Could you check a few things on this model? Use its own coordinates, in mm. Give positions to 0.01 mm unless a question says otherwise; leave off trailing zeros. Loops run counter-clockwise (first coordinate to the right, second up) from the corner with the lowest first, then second, coordinate; pieces in that order, holes last. Notation, with made-up numbers: M -22,77.5 L 13,77.5 A30 ccw 13,100.5 Z; hole C 59.25,71 d11. An arc over 180 degrees is marked long. Answer in a Markdown table with one row per item. Add a question column.
1. If we section it at D-D on x = -16.5: List the corners of the cut face in (y, z) for me.
2. If we section it at B-B on x = 0: List the corners of the cut face in (y, z) for me, then the cut area to 3 significant figures.
3. If we section it at A-A on z = 0: List the corners of the cut face in (x, y) for me.
4. If we section it at C-C on y = 1.6: Count the separate pieces of the cut face and the enclosed holes in it, then the cut area to 3 significant figures.
5. I need wall thicknesses on line 1 along Z through (x, y) = (0, 1.3); line 2 along Z through (x, y) = (-22.5, 0.95); line 3 along Z through (x, y) = (-7.5, 2). Which ranges of each line are inside material? Lowest first, please. Write a range as from..to.
6. I'm going to push flat-ended pins straight in: pin 1 Ø2 at (x, z) = (8.13, -22.27) entering from -Y; pin 2 Ø1 at (x, y) = (-11, 2.5) entering from -Z. Where does each tip first touch, or does it pass through?
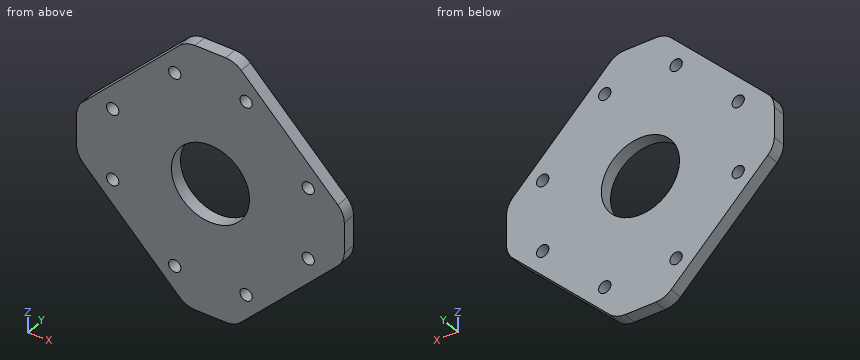
```python
from build123d import *

# Parameters (mm, degrees)
SKETCH1_R           = 8.9
SKETCH1_R_2         = 1.4
BOSS_EXTRUDE1_DEPTH = 3


with BuildPart() as part:
    # Sketch1 → Boss-Extrude1 (new body)
    with BuildSketch(Plane(origin=(0, 0, 0), x_dir=(1, 0, 0), z_dir=(0, 1, 0))):
        with BuildLine():
            Line((3.491378029, 30.5), (-3.491378029, 30.5))
            ThreePointArc((-3.491378029, 30.5), (-5.40479519, 30.119397663), (-7.026911935, 29.035533906))
            Line((-7.026911935, 29.035533906), (-29.035533906, 7.026911935))
            ThreePointArc((-29.035533906, 7.026911935), (-30.119397663, 5.40479519), (-30.5, 3.491378029))
            Line((-30.5, 3.491378029), (-30.5, -3.491378029))
            ThreePointArc((-30.5, -3.491378029), (-30.119397663, -5.40479519), (-29.035533906, -7.026911935))
            Line((-29.035533906, -7.026911935), (-7.026911935, -29.035533906))
            ThreePointArc((-7.026911935, -29.035533906), (-5.40479519, -30.119397663), (-3.491378029, -30.5))
            Line((-3.491378029, -30.5), (3.491378029, -30.5))
            ThreePointArc((3.491378029, -30.5), (5.40479519, -30.119397663), (7.026911935, -29.035533906))
            Line((7.026911935, -29.035533906), (29.035533906, -7.026911935))
            ThreePointArc((29.035533906, -7.026911935), (30.119397663, -5.40479519), (30.5, -3.491378029))
            Line((30.5, -3.491378029), (30.5, 3.491378029))
            ThreePointArc((30.5, 3.491378029), (30.119397663, 5.40479519), (29.035533906, 7.026911935))
            Line((29.035533906, 7.026911935), (7.026911935, 29.035533906))
            ThreePointArc((7.026911935, 29.035533906), (5.40479519, 30.119397663), (3.491378029, 30.5))
        make_face()
        Circle(SKETCH1_R, mode=Mode.SUBTRACT)
        with Locations((8.131727984, -22.273863607)):
            Circle(SKETCH1_R_2, mode=Mode.SUBTRACT)
        with Locations((-8.131727984, -22.273863607)):
            Circle(SKETCH1_R_2, mode=Mode.SUBTRACT)
        with Locations((-22.273863607, -8.131727984)):
            Circle(SKETCH1_R_2, mode=Mode.SUBTRACT)
        with Locations((22.273863607, -8.131727984)):
            Circle(SKETCH1_R_2, mode=Mode.SUBTRACT)
        with Locations((22.273863607, 8.131727984)):
            Circle(SKETCH1_R_2, mode=Mode.SUBTRACT)
        with Locations((8.131727984, 22.273863607)):
            Circle(SKETCH1_R_2, mode=Mode.SUBTRACT)
        with Locations((-8.131727984, 22.273863607)):
            Circle(SKETCH1_R_2, mode=Mode.SUBTRACT)
        with Locations((-22.273863607, 8.131727984)):
            Circle(SKETCH1_R_2, mode=Mode.SUBTRACT)
    extrude(amount=BOSS_EXTRUDE1_DEPTH)


solid = part.part
```
Results:
| question | item | result |
|---|---|---|
| 1 | outline | M 0,-19.56 L 3,-19.56 L 3,19.56 L 0,19.56 Z |
| 2 | outline | M 0,-30.5 L 3,-30.5 L 3,-8.9 L 0,-8.9 Z; M 0,8.9 L 3,8.9 L 3,30.5 L 0,30.5 Z |
| 2 | area | 130 mm2 |
| 3 | outline | M -30.5,0 L -8.9,0 L -8.9,3 L -30.5,3 Z; M 8.9,0 L 30.5,0 L 30.5,3 L 8.9,3 Z |
| 4 | separate pieces | 1 |
| 4 | enclosed holes | 9 |
| 4 | area | 2,170 mm2 |
| 5 | line 1 | -30.5..-8.9, 8.9..30.5 |
| 5 | line 2 | -13.56..-9.51, -6.75..6.75, 9.51..13.56 |
| 5 | line 3 | -28.56..-23.52, -21.02..-4.79, 4.79..21.02, 23.52..28.56 |
| 6 | pin 1 | through |
| 6 | pin 2 | z = -25.56 |
